Could you check a few things on this model? Use its own coordinates, in mm. Face numbers are marked on the shaded views. A direction names the side the tool comes from. Coordinates: 2 decimals unless noted, no trailing zeros. Loops run counter-clockwise (first coordinate to the right, second up) from the corner with the lowest first, then second, coordinate; pieces in that order, holes last.
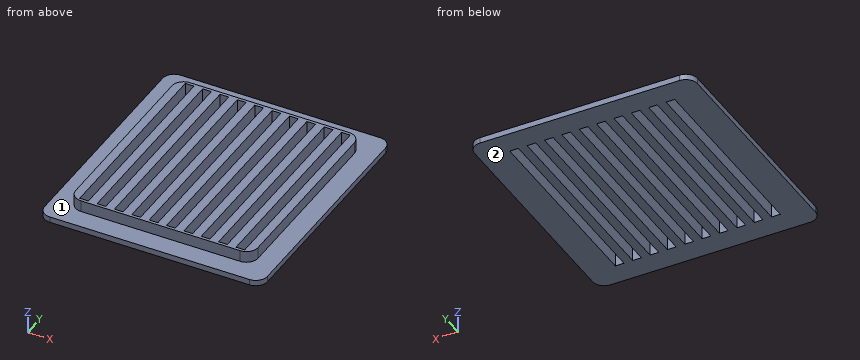
from build123d import *

# Parameters (mm, degrees)
F0_W     = 77
F0_H     = 84
F1_DEPTH = 2
F2_W     = 63
F2_H     = 70
F3_DEPTH = 4
F4_W     = 3
F4_H     = 68
F5_DEPTH = 6.001
F6_R     = 4


with BuildPart() as f1:
    # F0 (on Top) → F1 (new body)
    with BuildSketch(Plane.XY):
        Rectangle(F0_W, F0_H)
    extrude(amount=F1_DEPTH)

    # F2 (on face) → F3 (join)
    with BuildSketch(Plane.XY.offset(2)):
        Rectangle(F2_W, F2_H)
    extrude(amount=F3_DEPTH)

    # F4 (on face) → F5 (cut, through all)
    with BuildSketch(Plane.XY.offset(6)):
        with Locations((3, 0)):
            Rectangle(F4_W, F4_H)
        with Locations((9, 0)):
            Rectangle(F4_W, F4_H)
        with Locations((15, 0)):
            Rectangle(F4_W, F4_H)
        with Locations((21, 0)):
            Rectangle(F4_W, F4_H)
        with Locations((27, 0)):
            Rectangle(F4_W, F4_H)
        with Locations((-3, 0)):
            Rectangle(F4_W, F4_H)
        with Locations((-9, 0)):
            Rectangle(F4_W, F4_H)
        with Locations((-15, 0)):
            Rectangle(F4_W, F4_H)
        with Locations((-21, 0)):
            Rectangle(F4_W, F4_H)
        with Locations((-27, 0)):
            Rectangle(F4_W, F4_H)
    extrude(amount=-F5_DEPTH, mode=Mode.SUBTRACT)

    # F6
    f6_edges = [f1.edges().sort_by_distance(p)[0] for p in [
        (-38.5, -42, 1),
        (-31.5, -35, 4),
        (31.5, -35, 4),
        (38.5, -42, 1),
        (-31.5, 35, 4),
        (-38.5, 42, 1),
        (31.5, 35, 4),
        (38.5, 42, 1),
    ]]
    fillet(f6_edges, radius=F6_R)


solid = f1.part
(1) Which directions (+Z, -Z, +X, -X, +Y, -Y) give clear straight access to the entire face, cutting with the end or side of a thin tool? Please do the marked faces 1 and 2.
Answers:
face 1: +Z
face 2: -Z, +X, -X, +Y, -Y
(2) Imagine slicing it at B-B, the plane x = 0.5. Write out the boundary of the cut face in (y, z).
Answers:
outline: (-42, 0) - (42, 0) - (42, 2) - (35, 2) - (35, 6) - (-35, 6) - (-35, 2) - (-42, 2) - close
(3) Imagine slicing it at A-A, the plane x = -9. Write out the boundary of the cut face in (y, z).
Answers:
outline: (-42, 0) - (-34, 0) - (-34, 6) - (-35, 6) - (-35, 2) - (-42, 2) - close; (34, 0) - (42, 0) - (42, 2) - (35, 2) - (35, 6) - (34, 6) - close
(4) Imagine slicing it at C-C, the plane y = 10.5. State how many separate pieces and enclosed holes the cut face has, and give its area (3 significant figures).
Answers:
separate pieces: 11
enclosed holes: 0
area: 226 mm2
(5) I need wall thicknesses on probe 1 along Y at (x, z) = (-4, 0.5); probe 2 along Y at (x, z) = (15.5, 2.25); probe 3 along Y at (x, z) = (-1, 3.9). Which ranges of each line are inside material? Lowest first, please.
Answers:
probe 1: y = -42 to -34, 34 to 42
probe 2: y = -35 to -34, 34 to 35
probe 3: y = -35 to 35
(6) For pin 1 (1.8 mm diameter, centred on y = 0, z = 3, fed in from -X); pin 2 (1 mm diameter, centred on y = -31, z = 4.5, fed in from +X); pin 3 (1.5 mm diameter, centred on x = 8.5, z = 3.5, fed in from -Y), each with a flat end and sliding along its axis, tell me the tip position at first contact or that it passes through.
Answers:
pin 1: stops at x = -31.5
pin 2: stops at x = 31.5
pin 3: stops at y = -35
